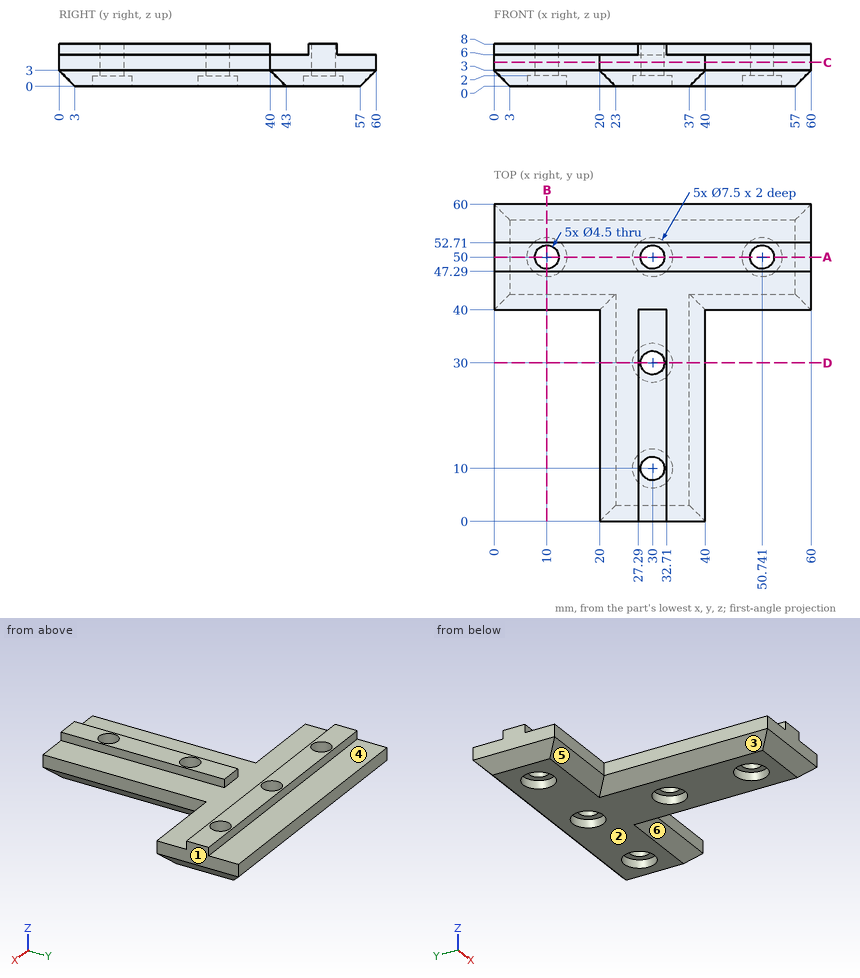
Geometry check sheet. Reference: drawing and pictorial views, mm from the part's lowest x, y, z. A direction names the side the tool comes from. Round coordinates to 2 decimals unless told otherwise and drop trailing zeros. Loops run counter-clockwise (first coordinate to the right, second up) from the corner with the lowest first, then second, coordinate; pieces in that order, holes last. Notation, with made-up numbers: (-36.75, 0) - (13.25, 0) arc R9 cw to (13.25, 4) - close; hole circle Ø3 at (65, 37.5). An arc over 180 degrees is marked (long way). Answer in a Markdown table with one row per item. Add a question column.
Q1. Section check D-D on y = 30. Enter the section's corners in (x, z).
Q2. Section check B-B on x = 10. Enter the section's corners in (y, z).
Q3. Section check C-C on z = 4.5. Enter the section's corners in (x, y), plus the area to 3 significant figures.
Q4. Gauge pin test, flat ends, axial feed: pin 1 (0.9 mm diameter, centred on y = 28, z = 4, fed in from +X); pin 2 (1.5 mm diameter, centred on y = 30.5, z = 4, fed in from -X); pin 3 (10 mm diameter, centred on x = 20.5, y = 24.5, fed in from +Z). Record the tip position at first contact, or that the pin passes through.
Q5. Section check A-A on y = 50. State how many separate pieces and enclosed holes the cut face has, plus the area to 3 significant figures.
Q6. Tool access check on the marked faces 4, 5 and 6. Record the directions out of +Z, -Z, +X, -X, +Y, -Y that give a thin tool (end or side, any length) a straight path to the whole face; none if there is none.
Q7. Release check for a two-part mould opening along X. For the marked faces 1, 2 and 3 record: pulls with the +X half, pulls with the -X half, needs draft (parallel to the pull), parting line crosses it, or undercut.
Q8. Material ranges on line 1 (Y direction, x = 30, z = 4.75); line 2 (X direction, y = 50, z = 0.8); line 3 (X direction, y = 50, z = 0.7), recorded low to high.
Found:
| question | item | result |
|---|---|---|
| 1 | outline | (20, 3) - (23, 0) - (26.25, 0) - (26.25, 2) - (27.75, 2) - (27.75, 8) - (27.29, 8) - (27.29, 6) - (20, 6) - close; (32.25, 2) - (33.75, 2) - (33.75, 0) - (37, 0) - (40, 3) - (40, 6) - (32.71, 6) - (32.71, 8) - (32.25, 8) - close |
| 2 | outline | (40, 3) - (43, 0) - (46.25, 0) - (46.25, 2) - (47.75, 2) - (47.75, 8) - (47.29, 8) - (47.29, 6) - (40, 6) - close; (52.25, 2) - (53.75, 2) - (53.75, 0) - (57, 0) - (60, 3) - (60, 6) - (52.71, 6) - (52.71, 8) - (52.25, 8) - close |
| 3 | outline | (0, 40) - (20, 40) - (20, 0) - (40, 0) - (40, 40) - (60, 40) - (60, 60) - (0, 60) - close; hole circle Ø4.5 at (10, 50); hole circle Ø4.5 at (30, 10); hole circle Ø4.5 at (30, 30); hole circle Ø4.5 at (30, 50); hole circle Ø4.5 at (50.74, 50) |
| 3 | area | 1,920 mm² |
| 4 | pin 1 | stops at x = 40 |
| 4 | pin 2 | stops at x = 20 |
| 4 | pin 3 | stops at z = 6 |
| 5 | separate pieces | 4 |
| 5 | enclosed holes | 0 |
| 5 | area | 345 mm² |
| 6 | face 4 | +Z, +X, -X, +Y |
| 6 | face 5 | -Z, -X, -Y |
| 6 | face 6 | -Z, +X, -Y |
| 7 | face 1 | pulls with the +X half |
| 7 | face 2 | needs draft |
| 7 | face 3 | pulls with the -X half |
| 8 | line 1 | y = 0 to 7.75, 12.25 to 27.75, 32.25 to 47.75, 52.25 to 60 |
| 8 | line 2 | x = 2.2 to 6.25, 13.75 to 26.25, 33.75 to 46.99, 54.49 to 57.8 |
| 8 | line 3 | x = 2.3 to 6.25, 13.75 to 26.25, 33.75 to 46.99, 54.49 to 57.7 |
